Part model, mm, in its own coordinate system. A direction names the side the tool comes from. Coordinates: 2 decimals unless noted, no trailing zeros. Loops run counter-clockwise (first coordinate to the right, second up) from the corner with the lowest first, then second, coordinate; pieces in that order, holes last. Notation, with made-up numbers: M -8.5,-4 L 21.5,-4 A25 ccw 21.5,11 Z; hole C 56,-8.75 d8. An arc over 180 degrees is marked long. Use CSV: the item, a comma, the result in double quotes. Start each with the question number.
from build123d import *

# Parameters (mm, degrees)
SKETCH1_R           = 18
SKETCH1_R_2         = 8
BOSS_EXTRUDE1_DEPTH = 8
SKETCH2_R           = 8
SKETCH2_R_2         = 6
BOSS_EXTRUDE2_DEPTH = 1.6
SKETCH3_W           = 40
SKETCH3_H           = 20
CUT_EXTRUDE1_DEPTH  = 9
CUT_EXTRUDE2_REACH  = 19
SKETCH5_R           = 1.6
CUT_EXTRUDE3_REACH  = 27
CUT_EXTRUDE3_START  = -8
SKETCH6_R           = 3


with BuildPart() as part:
    # Sketch1 → Boss-Extrude1 (new body)
    with BuildSketch(Plane(origin=(0, 0, 0), x_dir=(1, 0, 0), z_dir=(0, 1, 0))):
        Circle(SKETCH1_R)
        Circle(SKETCH1_R_2, mode=Mode.SUBTRACT)
    extrude(amount=BOSS_EXTRUDE1_DEPTH)

    # Sketch2 → Boss-Extrude2 (add)
    with BuildSketch(Plane(origin=(0, 0, 0), x_dir=(1, 0, 0), z_dir=(0, 1, 0))):
        Circle(SKETCH2_R)
        Circle(SKETCH2_R_2, mode=Mode.SUBTRACT)
    extrude(amount=BOSS_EXTRUDE2_DEPTH)

    # Sketch3 → Cut-Extrude1 (cut, through all)
    with BuildSketch(Plane(origin=(0, 8, 0), x_dir=(1, 0, 0), z_dir=(0, 1, 0))):
        with Locations((0, -9)):
            Rectangle(SKETCH3_W, SKETCH3_H)
    extrude(amount=-CUT_EXTRUDE1_DEPTH, mode=Mode.SUBTRACT)

    # Sketch5 → Cut-Extrude2 (cut, up to next)
    with BuildSketch(Plane.XY.offset(-1), mode=Mode.PRIVATE) as cut_extrude2_sk1:
        with Locations((-12.954727344, 4)):
            Circle(SKETCH5_R)
    cut_extrude2_tool1 = extrude(cut_extrude2_sk1.sketch, amount=-CUT_EXTRUDE2_REACH, mode=Mode.PRIVATE) & part.part
    add(cut_extrude2_tool1.solids().sort_by_distance((-12.954727, 4, -1))[0], mode=Mode.SUBTRACT)
    # Sketch5 → Cut-Extrude2 (cut, up to next)
    with BuildSketch(Plane.XY.offset(-1), mode=Mode.PRIVATE) as cut_extrude2_sk2:
        with Locations((12.954727344, 4)):
            Circle(SKETCH5_R)
    cut_extrude2_tool2 = extrude(cut_extrude2_sk2.sketch, amount=-CUT_EXTRUDE2_REACH, mode=Mode.PRIVATE) & part.part
    add(cut_extrude2_tool2.solids().sort_by_distance((12.954727, 4, -1))[0], mode=Mode.SUBTRACT)

    # Sketch6 → Cut-Extrude3 (cut, up to next)
    with BuildSketch(Plane.XY.offset(-1).offset(CUT_EXTRUDE3_START), mode=Mode.PRIVATE) as cut_extrude3_sk1:
        with Locations((-12.954727344, 4)):
            Circle(SKETCH6_R)
    cut_extrude3_tool1 = extrude(cut_extrude3_sk1.sketch, amount=-CUT_EXTRUDE3_REACH, mode=Mode.PRIVATE) & part.part
    add(cut_extrude3_tool1.solids().sort_by_distance((-12.954727, 4, -9))[0], mode=Mode.SUBTRACT)
    # Sketch6 → Cut-Extrude3 (cut, up to next)
    with BuildSketch(Plane.XY.offset(-1).offset(CUT_EXTRUDE3_START), mode=Mode.PRIVATE) as cut_extrude3_sk2:
        with Locations((12.954727344, 4)):
            Circle(SKETCH6_R)
    cut_extrude3_tool2 = extrude(cut_extrude3_sk2.sketch, amount=-CUT_EXTRUDE3_REACH, mode=Mode.PRIVATE) & part.part
    add(cut_extrude3_tool2.solids().sort_by_distance((12.954727, 4, -9))[0], mode=Mode.SUBTRACT)


solid = part.part
1. Slice it at C-C, the plane x = 12. List the corners of the cut face in (y, z), and give its area (3 significant figures).
2. Pin check, flat tips, straight feed: pin 1 (2 mm diameter, centred on x = 0, y = 2.5, fed in from +Z); pin 2 (3 mm diameter, centred on x = 12.95, y = 4, fed in from +Z); pin 3 (1 mm diameter, centred on x = 7, y = 1.5, fed in from -Z); pin 4 (2 mm diameter, centred on y = 5, z = -11, fed in from +X). Stop position of each tip, or through.
3. Tool access for faces 1 (the face through (13, 2, -1)), 2 (the face through (-9.957, 3.889, -11.29)), 3 (the face through (0, 5, -8)): list every direction of +Z, -Z, +X, -X, +Y, -Y with a clear straight run to the whole face (end or side of a thin tool).
4. Slice it at D-D, the plane x = 0. List the corners of the cut face in (y, z), and give its area (3 significant figures).
5. Slice it at A-A, the plane z = -4.5. List the corners of the cut face in (x, y).
6. Two-plate mould, pull along Y, no slides. Class faces 4 (the face through (-12, 2, -1)), 5 (the face through (-14.224, 3.026, -4.944)), 6 (the face through (9.957, 4.111, -11.29)), 7 (the face through (-0.6, 1.6, -6.3)): pulls with the +Y half, pulls with the -Y half, needs draft (parallel to the pull), parting line crosses it, or undercut.
7. Wall check: probe 1 along X at (y, z) = (3.5, -1.75); probe 2 along X at (y, z) = (4, -10.8); probe 3 along Y at (x, z) = (-6, -4.5). Give the ranges that are in metal, low to high.
8. Slice it at B-B, the plane y = 4. List the corners of the cut face in (x, z).
Found:
1,outline,"M 0,-13.42 L 1.16,-13.42 L 1.16,-9 L 2.72,-9 L 2.72,-1 L 0,-1 Z; M 5.28,-9 L 6.84,-9 L 6.84,-13.42 L 8,-13.42 L 8,-1 L 5.28,-1 Z"
1,area,"53.7 mm^2"
2,pin 1,"z = -5.98"
2,pin 2,"through"
2,pin 3,"z = -16.79"
2,pin 4,"x = 10.72"
3,face 1,"+Z, +X, -X, +Y, -Y"
3,face 2,"-Z"
3,face 3,"+Z, +Y"
4,outline,"M 0,-18 L 8,-18 L 8,-8 L 1.6,-8 L 1.6,-6 L 0,-6 Z"
4,area,"83.2 mm^2"
5,outline,"M -17.43,0 L -3.97,0 L -3.97,1.6 L -6.61,1.6 L -6.61,8 L -17.43,8 Z; M 3.97,0 L 17.43,0 L 17.43,8 L 6.61,8 L 6.61,1.6 L 3.97,1.6 Z; hole C -12.95,4 d3.2; hole C 12.95,4 d3.2"
6,face 4,"needs draft"
6,face 5,"undercut"
6,face 6,"undercut"
6,face 7,"pulls with the +Y half"
7,probe 1,"-17.91 to -14.47, -11.43 to -7.81, 7.81 to 11.43, 14.47 to 17.91"
7,probe 2,"-9.95 to 9.95"
7,probe 3,"0 to 1.6"
8,outline,"M -17.97,-1 A18 ccw -15.59,-9 L -14.55,-9 L -14.55,-1 Z; M -11.35,-9 L -9.95,-9 L -9.95,-15 A18 ccw 9.95,-15 L 9.95,-9 L 11.35,-9 L 11.35,-1 L 7.94,-1 A8 cw -7.94,-1 L -11.35,-1 Z; M 14.55,-9 L 15.59,-9 A18 ccw 17.97,-1 L 14.55,-1 Z"
